Can you work these out from the drawing? Everything is in mm from the part's minimum corner. A direction names the side the tool comes from. Coordinates: 2 decimals unless noted, no trailing zeros. Write each loop counter-clockwise with the first axis right and the second up, starting at its lowest first coordinate (ties: lowest second). Pieces come first, ordered by that corner, then holes. Notation, with made-up numbers: M 77,-37 L 110,-37 A19 ccw 110,-24 Z; hole C 17.25,-23 d11. An arc over 180 degrees is marked long. Answer as a JSON object with one key per item and string values. Group by question number.
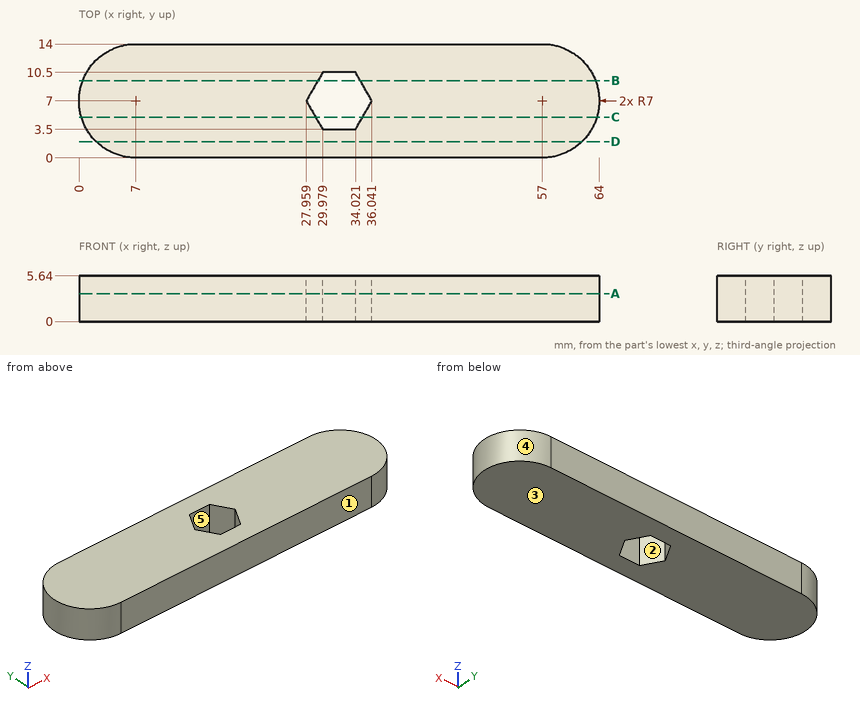
Q1. Please list where these lines run through material, in increasing order: L1, parallel to Y at x = 34, z = 0.5; L2, parallel to X at y = 9.5, z = 3.95; L3, parallel to X at y = 4, z = 2.7 (1 decimal).
Q2. On a 3-axis mill with a long thin cutter (end or side, diameter ignored), from which of +Z, -Z, +X, -X, +Y, -Y can I reach the whole of each face in a straight line? I mean the marked faces 1 and 2. Say none if no direction works.
Q3. If we section it at D-D on y = 2: List the corners of the cut face in (x, z) for me.
Q4. We'd pull the mould along Y, two halves only. Please class the marked faces 3, 4 and 5: pulls with the +Y half, pulls with the -Y half, needs draft (parallel to the pull), parting line crosses it, or undercut.
Q5. Will these pins go through, and if not, where does the flat tip stop? pin 1 (8 mm diameter, centred on x = 12.5, y = 11.5, fed in from -Z); pin 2 (2 mm diameter, centred on y = 11, z = 0.5, fed in from -X) (1 decimal); pin 3 (1 mm diameter, centred on y = 4.5, z = 4.5, fed in from -X).
Q6. If we section it at C-C on y = 5: List the corners of the cut face in (x, z) for me, and give its area (3 significant figures).
Q7. If we section it at A-A on z = 3.45: List the corners of the cut face in (x, y) for me.
Q8. If we section it at B-B on y = 9.5: List the corners of the cut face in (x, z) for me.
Reply:
{
 "1": {"L1": "0 to 3.5, 10.5 to 14", "L2": "0.46 to 29.4, 34.6 to 63.54", "L3": "0.7 to 29.7, 34.3 to 63.3"},
 "2": {"face 1": "+Z, -Z, +X, -X, -Y", "face 2": "+Z, -Z"},
 "3": {"outline": "M 2.1,0 L 61.9,0 L 61.9,5.64 L 2.1,5.64 Z"},
 "4": {"face 3": "needs draft", "face 4": "parting line crosses it", "face 5": "undercut"},
 "5": {"pin 1": "z = 0", "pin 2": "x = 0.7", "pin 3": "x = 0.29"},
 "6": {"outline": "M 0.29,0 L 29.11,0 L 29.11,5.64 L 0.29,5.64 Z; M 34.89,0 L 63.71,0 L 63.71,5.64 L 34.89,5.64 Z", "area": "325 mm^2"},
 "7": {"outline": "M 7,0 L 57,0 A7 ccw 57,14 L 7,14 A7 ccw Z; hole M 27.96,7 L 29.98,3.5 L 34.02,3.5 L 36.04,7 L 34.02,10.5 L 29.98,10.5 Z"},
 "8": {"outline": "M 0.46,0 L 29.4,0 L 29.4,5.64 L 0.46,5.64 Z; M 34.6,0 L 63.54,0 L 63.54,5.64 L 34.6,5.64 Z"}
}
